For this review, take the finished solid that the model builds, in its own axes (mm). A direction names the side the tool comes from. Give positions to 0.01 mm unless a question says otherwise; leave off trailing zeros. Loops run counter-clockwise (first coordinate to the right, second up) from the corner with the lowest first, then second, coordinate; pieces in that order, holes last.
```python
from build123d import *

# Parameters (mm, degrees)
SKETCH_1_R             = 5
EXTRUDE_1_DEPTH        = 150
CUT_EXTRUDE_1_DEPTH    = 3
SKETCH_3_R             = 5
EXTRUDE_2_DEPTH        = 150
CUT_EXTRUDE_2_DEPTH    = 3
EXTRUDE_START          = 80
SKETCH_5_R             = 5
EXTRUDE_4_DEPTH        = 80
PATTERN_LINEAR_2_COUNT = 2
PATTERN_LINEAR_2_PITCH = 65


with BuildPart() as part:
    # 草图1 → 凸台-拉伸1 (new body)
    with BuildSketch(Plane(origin=(0, 0, 0), x_dir=(0, 0, -1), z_dir=(1, 0, 0))):
        Circle(SKETCH_1_R)
    extrude(amount=EXTRUDE_1_DEPTH)

    # 草图2 → 切除-拉伸1 (cut)
    with BuildSketch(Plane(origin=(0, 5, 0), x_dir=(1, 0, 0), z_dir=(0, 1, 0))):
        with BuildLine():
            Line((23, 3), (37, 3))
            ThreePointArc((37, 3), (40, 0), (37, -3))
            Line((37, -3), (23, -3))
            ThreePointArc((23, -3), (20, 0), (23, 3))
        make_face()
    cut_extrude_1 = extrude(amount=-CUT_EXTRUDE_1_DEPTH, mode=Mode.SUBTRACT)

    # 草图3 → 凸台-拉伸2 (add)
    with BuildSketch(Plane(origin=(150, 0, 0), x_dir=(0, 0, -1), z_dir=(1, 0, 0))):
        Circle(SKETCH_3_R)
    extrude(amount=EXTRUDE_2_DEPTH)

    # 草图4 → 切除-拉伸2 (cut)
    with BuildSketch(Plane(origin=(0, 5, 0), x_dir=(1, 0, 0), z_dir=(0, 1, 0))):
        with BuildLine():
            Line((243, 3), (257, 3))
            ThreePointArc((257, 3), (260, 0), (257, -3))
            Line((257, -3), (243, -3))
            ThreePointArc((243, -3), (240, 0), (243, 3))
        make_face()
    extrude(amount=-CUT_EXTRUDE_2_DEPTH, mode=Mode.SUBTRACT)

    # 草图5 → 凸台-拉伸4 (add)
    with BuildSketch(Plane.ZY.offset(EXTRUDE_START)):
        Circle(SKETCH_5_R)
    extrude(amount=-EXTRUDE_4_DEPTH)

    # 阵列(线性)2: 切除-拉伸1 ×2
    with Locations(*[(-i * PATTERN_LINEAR_2_PITCH, 0, 0) for i in range(1, PATTERN_LINEAR_2_COUNT)]):
        add(cut_extrude_1, mode=Mode.SUBTRACT)


solid = part.part
```
Item 1: For L1, parallel to X at y = 3, z = 0.75; L2, parallel to X at y = 3.5, z = 2.25; L3, parallel to Y at x = 203, z = -0.75, list the stretches that pass through material, from the lowest coordinate up.
Answer:
L1: x = -80 to -44.9, -25.1 to 20.1, 39.9 to 240.1, 259.9 to 300
L2: x = -80 to -43.98, -26.02 to 21.02, 38.98 to 241.02, 258.98 to 300
L3: y = -4.94 to 4.94
Item 2: The part is to be moulded in two halves that separate along Z. For faces 3 (the flat face through (250, 2, 0)), 4 (the flat face through (-80, 0, 0)), say which applies: released by +Z, released by -Z, zero draft, split by the parting line, or undercut.
Answer:
face 3: undercut
face 4: zero draft
Item 3: Take a section at C-C on y = -3. Give the boundary of the cut face in (x, z).
Answer:
outline: (-80, -4) - (300, -4) - (300, 4) - (-80, 4) - close
Item 4: Take a section at B-B on z = 0.25. Give the boundary of the cut face in (x, y).
Answer:
outline: (-80, -4.99) - (300, -4.99) - (300, 4.99) - (259.99, 4.99) - (259.99, 2) - (240.01, 2) - (240.01, 4.99) - (39.99, 4.99) - (39.99, 2) - (20.01, 2) - (20.01, 4.99) - (-25.01, 4.99) - (-25.01, 2) - (-44.99, 2) - (-44.99, 4.99) - (-80, 4.99) - close
Item 5: Take a section at D-D on x = 29. Give the boundary of the cut face in (y, z), and give its area (3 significant figures).
Answer:
outline: (2, -3) - (2, 3) - (4, 3) arc R5 ccw (long way) to (4, -3) - close
area: 62.5 mm2
Item 6: Clearance check with flat-ended pins moving along their axes: pin 1 Ø3 at (x, y) = (138.5, 3) entering from +Z; pin 2 Ø1 at (x, y) = (-32.5, 2.5) entering from -Z; pin 3 Ø1.6 at (x, y) = (27, 3) entering from +Z. State where each tip first meets the part, or that it passes through.
Answer:
pin 1: stops at z = 4.77
pin 2: stops at z = -4.58
pin 3: stops at z = 4.49
Item 7: Take a section at A-A on x = 95.5. Give the boundary of the cut face in (y, z).
Answer:
outline: circle Ø10 at (0, 0)
Item 8: Tool access review of faces 1 (the flat face through (300, 0, 0)), 2 (the flat face through (-35, 2, 0)): name each direction out of +Z, -Z, +X, -X, +Y, -Y from which nothing blocks a thin tool from reaching the whole face with its end or side.
Answer:
face 1: +Z, -Z, +X, +Y, -Y
face 2: +Y
